Autodesk Inventor part; units mm, degrees
ref_plane "YZ Plane" through (0, 0, 0) normal (1, 0, 0) x (0, 1, 0)
ref_plane "XZ Plane" through (0, 0, 0) normal (0, 1, 0) x (-1, 0, 0)
ref_plane "XY Plane" through (0, 0, 0) normal (0, 0, 1) x (1, 0, 0)
sketch "スケッチ1" plane through (0, 0, 0) normal (0, 0, 1) x (1, 0, 0)
  line L0 (-20, -30) -> (20, -30)
  line L1 (20, -30) -> (20, 30)
  line L2 (20, 30) -> (-20, 30)
  line L3 (-20, 30) -> (-20, -30)
  line L4 (-20, -30) -> (20, 30) construction
  line L5 (20, -30) -> (-20, 30) construction
  line L6 (-17.7, 27.7) -> (17.7, 27.7)
  line L7 (17.7, 27.7) -> (17.7, -27.7)
  line L8 (17.7, -27.7) -> (-17.7, -27.7)
  line L9 (-17.7, -27.7) -> (-17.7, 27.7)
  point P0 (0, 0)
  dimension "d0" = 40
  dimension "d1" = 60
  dimension "d2" = 2.3
extrude "押し出し1" add sketch "スケッチ1" along normal mid plane 60
chamfer "面取り1" distance 60 angle 45 1 edges at (0, -30, -30)
sketch "スケッチ2" plane through (-20, 30, 30) normal (0, 1, 0) x (1, 0, 0)
  point P0 (20, 30)
  point P1 (20, 30)
hole "穴1" at (0, 30, 0) direction (0, -1, 0) diameter 15 depth 8 tip angle 118
sketch "スケッチ4" plane through (-20, 30, 30) normal (0, 1, 0) x (1, 0, 0)
  line L0 (0, 0) -> (40, 0)
  line L1 (40, 0) -> (40, 15)
  line L2 (40, 15) -> (0, 15)
  line L3 (0, 15) -> (0, 0)
  point P0 (20, 30)
  dimension "d15" = 40
  dimension "d16" = 15
extrude "押し出し2" cut sketch "スケッチ4" against normal blind 80
properties part number "車軸受け2"
Verification items for the finished model (mm, model axes). A direction names the side the tool comes from. Give positions to 0.01 mm unless a question says otherwise; leave off trailing zeros. Loops run counter-clockwise (first coordinate to the right, second up) from the corner with the lowest first, then second, coordinate; pieces in that order, holes last.
1. Release check for a two-part mould opening along X. For faces 1 (the cylindrical face through (-0.33, 28.834, -7.493)), 2 (the flat face through (-20, 18, 2)), 3 (the flat face through (-17.7, 16, 3)), 4 (the flat face through (20, 17, 2)) record: +X half, -X half, draft (parallel to the pull), parting line (faces both ways), or undercut.
Derived:
face 1: undercut
face 2: -X half
face 3: undercut
face 4: +X half
2. Cross-section at D-D on z = -5. Record the cut outline in (x, y).
Derived:
outline: (-20, 5) - (-17.7, 5) - (-17.7, 27.7) - (-5.59, 27.7) - (-5.59, 30) - (-20, 30) - close; (5.59, 27.7) - (17.7, 27.7) - (17.7, 5) - (20, 5) - (20, 30) - (5.59, 30) - close
3. Cross-section at B-B on x = 0. Record the cut outline in (y, z), and give its area (3 significant figures).
Derived:
outline: (27.7, -27.7) - (30, -30) - (30, -7.5) - (27.7, -7.5) - close; (27.7, 7.5) - (30, 7.5) - (30, 15) - (27.7, 15) - close
area: 66.4 mm2
4. Go/stop test with a flat-tipped pin: P1, Ø10.5, axis at x = -4.5, z = -13, coming from the -Y side. Record where the tip stops, or that it passes through.
Derived:
P1: stops at y = 27.7
5. Cross-section at A-A on y = 25.5. Record the cut outline in (x, z).
Derived:
outline: (-20, -25.5) - (-17.7, -25.5) - (-17.7, 15) - (-20, 15) - close; (17.7, -25.5) - (20, -25.5) - (20, 15) - (17.7, 15) - close
6. Material ranges on probe 1 along X at (y, z) = (28.85, 0); probe 2 along X at (y, z) = (10, -9.5); probe 3 along Y at (x, z) = (-11, -17), recorded low to high.
Derived:
probe 1: x = -20 to -7.5, 7.5 to 20
probe 2: x = -20 to -17.7, 17.7 to 20
probe 3: y = 27.7 to 30
7. Cross-section at C-C on z = 0. Record the cut outline in (x, y).
Derived:
outline: (-20, 0) - (-17.7, 0) - (-17.7, 27.7) - (-7.5, 27.7) - (-7.5, 30) - (-20, 30) - close; (7.5, 27.7) - (17.7, 27.7) - (17.7, 0) - (20, 0) - (20, 30) - (7.5, 30) - close
8. Tool access check on faces 5 (the flat face through (18, 13, 15)), 6 (the flat face through (4, 27.7, -7)). Record the directions out of +Z, -Z, +X, -X, +Y, -Y that give a thin tool (end or side, any length) a straight path to the whole face; none if there is none.
Derived:
face 5: +Z, +X, -X, +Y, -Y
face 6: +Z, -Z, -Y
